Check sheet for the modelled part. Datum: model origin and axes. Units: mm. A direction names the side the tool comes from. Round coordinates to 2 decimals unless told otherwise and drop trailing zeros. Write each loop counter-clockwise with the first axis right and the second up, starting at its lowest first coordinate (ties: lowest second). Pieces come first, ordered by that corner, then holes.
Item 1: Section check B-B, the plane y = 3. Record the cut outline in (x, z) (3 decimals).
Item 2: Material ranges on line 1 along Z through (x, y) = (-19, -1.5); line 2 along Y through (x, z) = (-20, 11.75) (3 decimals), recorded low to high.
Item 3: Release check for a two-part mould opening along X. For faces 1 (the flat face through (-25.4, 0, 6)), 2 (the flat face through (0, 0, 0)), 3 (the flat face through (-22.225, 0, 12)) record: pulls with the +X half, pulls with the -X half, needs draft (parallel to the pull), parting line crosses it, or undercut.
Item 4: Set-up check for faces 4 (the flat face through (25.4, 0, 6)), 5 (the flat face through (-11, 1, 11.9)): record each of +Z, -Z, +X, -X, +Y, -Y from which the full face is reachable in a straight line by a thin tool's end or side.
Item 5: Section check D-D, the plane y = 0. Record the cut outline in (x, z) (3 decimals), plus the area to 3 significant figures.
from build123d import *

# Parameters (mm, degrees)
F0_W        = 50.8
F0_H        = 25.4
F1_DEPTH    = 12.7
F2_W        = 19.05
F2_H        = 19.05
F2_W_2      = 13.97
F2_H_2      = 13.97
F2_W_3      = 8.89
F2_H_3      = 8.89
F2_W_4      = 3.81
F2_H_4      = 3.81
F3_DEPTH    = 1
F4_DEPTH    = 1.25
F5_DEPTH    = 1.35
F6_SIZE2    = 0.24999
F6_SIZE     = 0.24999
F7_T4_DEPTH = 16.0483871792
F8_W        = 3.81
F8_H        = 3.81
F8_R        = 1.5
F9_DEPTH    = 0.8


# Not quite as in the source:
# - a fillet or chamfer that OpenCascade refuses, or shapes differently, is made with other operations: its cross-section is extruded or revolved along the edge and cut away or added
# - a fillet or chamfer is up to 0.001 mm smaller than in the source, because OpenCascade refuses the exact size


with BuildPart() as f1:
    # F0 (on Top) → F1 (new body)
    with BuildSketch(Plane.XY):
        Rectangle(F0_W, F0_H)
    extrude(amount=F1_DEPTH)

    # F2 (on face) → F3 (cut)
    with BuildSketch(Plane.XY.offset(12.7)):
        with Locations((-12.7, 0)):
            Rectangle(F2_W, F2_H)
        with Locations((-12.7, 0)):
            Rectangle(F2_W_2, F2_H_2, mode=Mode.SUBTRACT)
        with Locations((-12.7, 0)):
            Rectangle(F2_W_2, F2_H_2)
        with Locations((-12.7, 0)):
            Rectangle(F2_W_3, F2_H_3, mode=Mode.SUBTRACT)
        with Locations((-12.7, 0)):
            Rectangle(F2_W_3, F2_H_3)
        with Locations((-12.7, 0)):
            Rectangle(F2_W_4, F2_H_4, mode=Mode.SUBTRACT)
    extrude(amount=-F3_DEPTH, mode=Mode.SUBTRACT)

    # F2 (on face) → F4 (cut)
    with BuildSketch(Plane.XY.offset(12.7)):
        with Locations((-12.7, 0)):
            Rectangle(F2_W_2, F2_H_2)
        with Locations((-12.7, 0)):
            Rectangle(F2_W_3, F2_H_3, mode=Mode.SUBTRACT)
    extrude(amount=-F4_DEPTH, mode=Mode.SUBTRACT)

    # F2 (on face) → F5 (cut)
    with BuildSketch(Plane.XY.offset(12.7)):
        with Locations((-12.7, 0)):
            Rectangle(F2_W_3, F2_H_3)
        with Locations((-12.7, 0)):
            Rectangle(F2_W_4, F2_H_4, mode=Mode.SUBTRACT)
    extrude(amount=-F5_DEPTH, mode=Mode.SUBTRACT)

    # F6 (size 0.25 and 0.25 in the source; OpenCascade refuses exactly that, so slightly less here)
    f6_edges = [f1.edges().sort_by_distance(p)[0] for p in [
        (-12.7, 6.985, 11.45),
    ]]
    chamfer(f6_edges, length=F6_SIZE, length2=F6_SIZE2)

    # F7: chamfer of 0.45 x 0.2598076211 on 1 edges, made by hand


with BuildPart() as f7_tool2:
    # F7_s3 → F7_t4 (new body)
    with BuildSketch(Plane.XZ.offset(-7.8991985896)):
        Polygon((-19.235, 11.45), (-19.685, 11.7098076211), (-19.685, 11.45), align=None)
    extrude(amount=F7_T4_DEPTH)

    split(bisect_by=Plane.XY.offset(11.7), keep=Keep.BOTTOM)


with BuildPart() as f1_1:
    add(f1.part)

    # F7_t1: union F7_tool2
    add(f7_tool2.part)

    # F8 (on face) → F9 (cut)
    with BuildSketch(Plane.XY.offset(12.7)):
        with Locations((-12.7, 0)):
            Rectangle(F8_W, F8_H)
        with Locations((-12.7, 0)):
            Circle(F8_R, mode=Mode.SUBTRACT)
    extrude(amount=-F9_DEPTH, mode=Mode.SUBTRACT)


solid = f1_1.part
Values found:
1. outline: (-25.4, 0) - (25.4, 0) - (25.4, 12.7) - (-3.175, 12.7) - (-3.175, 11.7) - (-5.715, 11.7) - (-5.715, 11.45) - (-8.255, 11.45) - (-8.255, 11.35) - (-17.145, 11.35) - (-17.145, 11.45) - (-19.235, 11.45) - (-19.668, 11.7) - (-22.225, 11.7) - (-22.225, 12.7) - (-25.4, 12.7) - close
2. line 1: z = 0 to 11.45
2. line 2: y = -12.7 to -9.525, 9.525 to 12.7
3. face 1: pulls with the -X half
3. face 2: needs draft
3. face 3: undercut
4. face 4: +Z, -Z, +X, +Y, -Y
4. face 5: +Z
5. outline: (-25.4, 0) - (25.4, 0) - (25.4, 12.7) - (-3.175, 12.7) - (-3.175, 11.7) - (-5.715, 11.7) - (-5.715, 11.45) - (-8.255, 11.45) - (-8.255, 11.35) - (-10.795, 11.35) - (-10.795, 11.9) - (-11.2, 11.9) - (-11.2, 12.7) - (-14.2, 12.7) - (-14.2, 11.9) - (-14.605, 11.9) - (-14.605, 11.35) - (-17.145, 11.35) - (-17.145, 11.45) - (-19.235, 11.45) - (-19.668, 11.7) - (-22.225, 11.7) - (-22.225, 12.7) - (-25.4, 12.7) - close
5. area: 626 mm2
